Autodesk Inventor part; units mm, degrees
ref_plane "YZ Plane" through (0, 0, 0) normal (1, 0, 0) x (0, 1, 0)
ref_plane "XZ Plane" through (0, 0, 0) normal (0, 1, 0) x (-1, 0, 0)
ref_plane "XY Plane" through (0, 0, 0) normal (0, 0, 1) x (1, 0, 0)
sketch "Sketch1" plane through (0, 0, 0) normal (0, 0, 1) x (1, 0, 0)
  line L0 (0, 0) -> (0, 15) construction
  line L1 (0, 15) -> (40, 15) construction
  line L2 (40, 15) -> (40, 4)
  line L3 (40, 4) -> (15, 4)
  line L4 (15, 4) -> (15, 0)
  line L5 (15, 0) -> (0, 0)
  line L6 (0, 7) -> (37, 7)
  line L7 (37, 7) -> (37, 15)
  line L8 (37, 15) -> (40, 15)
  line L9 (0, 7) -> (0, 0)
  dimension "d0" = 4
  dimension "d1" = 15
  dimension "d2" = 15
  dimension "d5" = 3
  dimension "d6" = 3
  dimension "d12" = 40
extrude "Extrusion1" add sketch "Sketch1" along normal blind 40
sketch "Sketch2" plane through (0, 0, 0) normal (0, -1, 0) x (1, 0, 0)
  line L0 (0, 0) -> (0, 40)
  line L1 (15, 0) -> (15, 40)
  line L2 (0, 20) -> (15, 20) construction
  line L3 (0, 33) -> (15, 33) construction
  arc A0 (2, 34) -> (2, 32) centre (2, 33) ccw
  arc A1 (13, 32) -> (13, 34) centre (13, 33) ccw
  line L4 (2, 34) -> (13, 34)
  line L5 (2, 32) -> (13, 32)
  line L6 (0, 7) -> (15, 7) construction
  arc A2 (2, 8) -> (2, 6) centre (2, 7) ccw
  arc A3 (13, 6) -> (13, 8) centre (13, 7) ccw
  line L7 (2, 6) -> (13, 6)
  line L8 (2, 8) -> (13, 8)
  dimension "d7" = 2
  dimension "d8" = 2
  dimension "d9" = 2
  dimension "d13" = 13
extrude "Extrusion2" cut sketch "Sketch2" against normal blind 30
properties part number "Guide"
The model under review builds one solid part; all positions refer to its coordinate system, in mm. A direction names the side the tool comes from. Give positions to 0.01 mm unless a question says otherwise; leave off trailing zeros. Write each loop counter-clockwise with the first axis right and the second up, starting at its lowest first coordinate (ties: lowest second). Pieces come first, ordered by that corner, then holes. Notation, with made-up numbers: (-32, -8.75) -> (-25, -8.75) arc R11 cw to (-25, -3.75) -> close; hole circle Ø10 at (-27, 77). An arc over 180 degrees is marked (long way). Answer in a Markdown table with one row per item.
1) For L1, parallel to Z at x = 13, y = 5; L2, parallel to Y at x = 12, z = 13.5; L3, parallel to X at y = 11, z = 12.5, list the stretches that pass through material, from the lowest coordinate up. Write a range as [from, to].
Worked answers:
| item | result |
|---|---|
| L1 | [0, 6], [8, 32], [34, 40] |
| L2 | [0, 7] |
| L3 | [37, 40] |
2) Tool access review of faces 4 (the cylindrical face through (14, 3, 33)), 5 (the flat face through (0, 4, 20)), 6 (the flat face through (15, 2, 20)), 7 (the flat face through (18, 7, 20)), 8 (the flat face through (40, 10, 20)): name each direction out of +Z, -Z, +X, -X, +Y, -Y from which nothing blocks a thin tool from reaching the whole face with its end or side.
Worked answers:
| item | result |
|---|---|
| face 4 | +Y, -Y |
| face 5 | +Z, -Z, -X, +Y, -Y |
| face 6 | +Z, -Z, +X, -Y |
| face 7 | +Z, -Z, -X, +Y |
| face 8 | +Z, -Z, +X, +Y, -Y |
3) Clearance check with flat-ended pins moving along their axes: P1, Ø4, axis at x = 31, z = 4.5, coming from the +Y side; P2, Ø3, axis at y = 2, z = 27, coming from the +X side; P3, Ø4, axis at x = 9, y = 10, coming from the -Z side; P4, Ø12.5, axis at x = 33, z = 18, coming from the -Y side. State where each tip first meets the part, or that it passes through.
Worked answers:
| item | result |
|---|---|
| P1 | y = 7 |
| P2 | x = 15 |
| P3 | through |
| P4 | y = 4 |
4) Mouldability with a two-part tool opening along X and no side actions: class faces 1 (the flat face through (7, 3, 8)), 2 (the flat face through (37, 11, 20)), 3 (the flat face through (28, 4, 20)) as +X half, -X half, draft (parallel to the pull), parting line (faces both ways), or undercut.
Worked answers:
| item | result |
|---|---|
| face 1 | undercut |
| face 2 | -X half |
| face 3 | draft |
5) Add section C-C on z = 20. State the section outline as (x, y) points.
Worked answers:
| item | result |
|---|---|
| outline | (0, 0) -> (15, 0) -> (15, 4) -> (40, 4) -> (40, 15) -> (37, 15) -> (37, 7) -> (0, 7) -> close |
6) Add section B-B on x = 6.5. State the section outline as (y, z) points.
Worked answers:
| item | result |
|---|---|
| outline | (0, 0) -> (7, 0) -> (7, 6) -> (0, 6) -> close; (0, 8) -> (7, 8) -> (7, 32) -> (0, 32) -> close; (0, 34) -> (7, 34) -> (7, 40) -> (0, 40) -> close |
7) Add section A-A on z = 7. State the section outline as (x, y) points, plus the area to 3 significant figures.
Worked answers:
| item | result |
|---|---|
| outline | (0, 0) -> (1, 0) -> (1, 7) -> (0, 7) -> close; (14, 0) -> (15, 0) -> (15, 4) -> (40, 4) -> (40, 15) -> (37, 15) -> (37, 7) -> (14, 7) -> close |
| area | 113 mm² |
8) Add section D-D on y = 8. State the section outline as (x, z) points.
Worked answers:
| item | result |
|---|---|
| outline | (37, 0) -> (40, 0) -> (40, 40) -> (37, 40) -> close |
